from build123d import *

# Parameters (mm, degrees)
BOSS_EXTRUDE1_DEPTH    = 15
BOSS_EXTRUDE1_TAPER    = -25
SKETCH2_R              = 2
CUT_EXTRUDE1_DEPTH     = 17
CUT_EXTRUDE2_START     = -15
CUT_EXTRUDE2_OUTLINE_R = 32.062922841
CUT_EXTRUDE2_DEPTH     = 15
SKETCH1_3_R            = 1.7
CUT_EXTRUDE3_DEPTH     = 13


# Read off the part's stored shape, not the designer's step: Cut-Extrude2
with BuildPart() as part:
    # Sketch1 → Boss-Extrude1 (new body)
    with BuildSketch(Plane(origin=(0, 0, 0), x_dir=(1, 0, 0), z_dir=(0, 1, 0))):
        with BuildLine():
            ThreePointArc((6.4, 7.2), (0, 4), (-6.4, 7.2))
            ThreePointArc((-6.4, 7.2), (-8, 8), (-9.6, 7.2))
            add(Edge.make_bspline(
                [(-9.6, 7.2), (-15, 0), (-9.6, -7.2)],
                knots=[2.498091545, 2.498091545, 2.498091545, 3.785093762, 3.785093762, 3.785093762], degree=2, weights=[1, 0.8, 1]))
            ThreePointArc((-9.6, -7.2), (-8, -8), (-6.4, -7.2))
            ThreePointArc((-6.4, -7.2), (0, -4), (6.4, -7.2))
            ThreePointArc((6.4, -7.2), (8, -8), (9.6, -7.2))
            add(Edge.make_bspline(
                [(9.6, -7.2), (15, 0), (9.6, 7.2)],
                knots=[5.639684198, 5.639684198, 5.639684198, 6.926686416, 6.926686416, 6.926686416], degree=2, weights=[1, 0.8, 1]))
            ThreePointArc((9.6, 7.2), (8, 8), (6.4, 7.2))
        make_face()
    extrude(amount=-BOSS_EXTRUDE1_DEPTH, taper=BOSS_EXTRUDE1_TAPER)

    # Sketch2 → Cut-Extrude1 (cut)
    with BuildSketch(Plane.XZ.offset(15)):
        with Locations(Location((0, 0, 0), (0, 0, 270))):
            Circle(SKETCH2_R)
    extrude(amount=-CUT_EXTRUDE1_DEPTH, mode=Mode.SUBTRACT)

    # Cut-Extrude2 outline → Cut-Extrude2 (cut)
    with BuildSketch(Plane(origin=(0, 0, 0), x_dir=(1, 0, 0), z_dir=(0, 1, 0)).offset(CUT_EXTRUDE2_START)):
        Circle(CUT_EXTRUDE2_OUTLINE_R)
        with BuildLine():
            Line((9.015638796, -3.184455543), (7.265638796, -6.215544457))
            Line((7.265638796, -6.215544457), (12.898275754, -9.467548921))
            ThreePointArc((12.898275754, -9.467548921), (12.756358421, -9.657914881), (12.611631712, -9.846153846))
            ThreePointArc((12.611631712, -9.846153846), (9.812426671, -10.96836467), (7.45232783, -9.090909091))
            ThreePointArc((7.45232783, -9.090909091), (0, -4), (-7.45232783, -9.090909091))
            ThreePointArc((-7.45232783, -9.090909091), (-9.812426671, -10.96836467), (-12.611631712, -9.846153846))
            ThreePointArc((-12.611631712, -9.846153846), (-15.876287892, -1.985820424), (-14.648275754, 6.436460008))
            Line((-14.648275754, 6.436460008), (-9.015638796, 3.184455543))
            Line((-9.015638796, 3.184455543), (-7.265638796, 6.215544457))
            Line((-7.265638796, 6.215544457), (-12.898275754, 9.467548921))
            ThreePointArc((-12.898275754, 9.467548921), (-12.756358421, 9.657914881), (-12.611631712, 9.846153846))
            ThreePointArc((-12.611631712, 9.846153846), (-9.812426671, 10.96836467), (-7.45232783, 9.090909091))
            ThreePointArc((-7.45232783, 9.090909091), (0, 4), (7.45232783, 9.090909091))
            ThreePointArc((7.45232783, 9.090909091), (9.812426671, 10.96836467), (12.611631712, 9.846153846))
            ThreePointArc((12.611631712, 9.846153846), (15.876287892, 1.985820424), (14.648275754, -6.436460008))
            Line((14.648275754, -6.436460008), (9.015638796, -3.184455543))
        make_face(mode=Mode.SUBTRACT)
    extrude(amount=CUT_EXTRUDE2_DEPTH, mode=Mode.SUBTRACT)

    # Sketch1_3 → Cut-Extrude3 (cut)
    with BuildSketch(Plane(origin=(0, 0, 0), x_dir=(1, 0, 0), z_dir=(0, 1, 0))):
        with Locations(Location((9.5, 0, 0), (0, 0, 270))):
            Circle(SKETCH1_3_R)
        with Locations(Location((-9.5, 0, 0), (0, 0, 270))):
            Circle(SKETCH1_3_R)
    extrude(amount=-CUT_EXTRUDE3_DEPTH, mode=Mode.SUBTRACT)


solid = part.part
Model file for the job. Use its own axes, mm. A direction names the side the tool comes from. Round coordinates to 2 decimals unless told otherwise and drop trailing zeros. Order: outer loops, then holes, each group sorted by start corner. A loop starts at its lowest first (then second) coordinate and runs counter-clockwise, first axis right, second up.
(1) 3-axis set-ups, long thin cutter, end or side, ignore diameter. For faces 1 (the face through (7.84, -6.41, -0.37)), 2 (the face through (-9.4, -3.4, -9.3)), 3 (the face through (-8.15, -7.6, -4.68)): which of +Z, -Z, +X, -X, +Y, -Y reach the whole face in a straight line?
(2) Band-saw the part on A-A (x = 0). List the corners of the cut face in (y, z), then the cut area to 3 significant figures.
(3) Pin check, flat tips, straight feed: pin 1 (2 mm diameter, centred on x = 9.5, z = 0, fed in from +Y); pin 2 (2 mm diameter, centred on y = -2, z = -3.5, fed in from +X); pin 3 (3 mm diameter, centred on y = -2, z = 3, fed in from +X); pin 4 (2.5 mm diameter, centred on x = 0, z = 0, fed in from -Y). Stop position of each tip, or through.
(4) Drill centre lines: line 1 (X direction, y = -11.5, z = 0); line 2 (X direction, y = -12.25, z = 0.5); line 3 (X direction, y = -7.75, z = -4.75). Where is each one in solid material? Low to high.
(5) Band-saw the part on D-D (x = -4.5). List the corners of the cut face in (y, z).
(6) Band-saw the part on C-C (z = -5). Give the number of separate pieces and of enclosed holes in the cut face, then the cut area to 3 significant figures.
(7) Band-saw the part on B-B (y = -10.5). List the corners of the cut face in (x, z).
(8) Pull direction Z, two halves, no side cores. Call faces 4 (the face through (2, 0, 2)), 5 (the face through (10, -13, 0)), 6 (the face through (-9.09, -10.2, 10.77)), 7 (the face through (11.246, -9.272, 4.472)): released by +Z, released by -Z, zero draft, split by the parting line, or undercut.
Verdict:
1. face 1: +Y
1. face 2: -Z, +Y
1. face 3: +Y, -Y
2. outline: (-15, -4) - (0, -4) - (0, -2) - (-15, -2) - close; (-15, 2) - (0, 2) - (0, 4) - (-15, 4) - close
2. area: 60.0 mm2
3. pin 1: stops at y = -13
3. pin 2: stops at x = 13
3. pin 3: stops at x = 13.36
3. pin 4: passes through
4. line 1: x = -16 to -11.2, -7.8 to -2, 2 to 7.8, 11.2 to 16
4. line 2: x = -15.99 to -11.12, -7.88 to -1.94, 1.94 to 7.88, 11.12 to 15.99
4. line 3: x = -14.87 to -11.73, -8.11 to -3.38, 3.38 to 14.87
5. outline: (-15, -5.39) - (0, -5.39) - (0, 5.39) - (-15, 5.39) - close
6. separate pieces: 3
6. enclosed holes: 0
6. area: 242 mm2
7. outline: (-14.65, -6.44) - (-9.02, -3.18) - (-7.27, -6.22) - (-12.9, -9.47) arc R16 ccw to (-12.61, -9.85) arc R3 ccw to (-7.45, -9.09) arc R8 cw to (7.45, -9.09) arc R3 ccw to (12.61, -9.85) arc R16 ccw to (14.65, 6.44) - (9.02, 3.18) - (7.27, 6.22) - (12.9, 9.47) arc R16 ccw to (12.61, 9.85) arc R3 ccw to (7.45, 9.09) arc R8 cw to (-7.45, 9.09) arc R3 ccw to (-12.61, 9.85) arc R16 ccw to start; hole circle Ø3.4 at (-9.5, 0); hole circle Ø4 at (0, 0); hole circle Ø3.4 at (9.5, 0)
8. face 4: zero draft
8. face 5: undercut
8. face 6: released by +Z
8. face 7: undercut
